```python
from build123d import *

# Parameters (mm, degrees)
F1_ANGLE = 350


with BuildPart() as f1:
    # F0 (on Top) → F1 (revolve)
    with BuildSketch(Plane.XY):
        with BuildLine():
            Line((1.2065, 2.413), (17.792, 2.413))
            Line((17.792, 2.413), (17.792, 2.7178))
            Line((17.792, 2.7178), (1.2065, 2.7178))
            ThreePointArc((1.2065, 2.7178), (0.568902, 2.981902), (0.3048, 3.6195))
            Line((0.3048, 3.6195), (0.3048, 5.3815))
            Line((0.3048, 5.3815), (0, 5.3815))
            Line((0, 5.3815), (0, 3.6195))
            ThreePointArc((0, 3.6195), (0.353376, 2.766376), (1.2065, 2.413))
        make_face()
    revolve(axis=Axis((8.896, 0, 0), (1, 0, 0)), revolution_arc=F1_ANGLE)


solid = f1.part
```
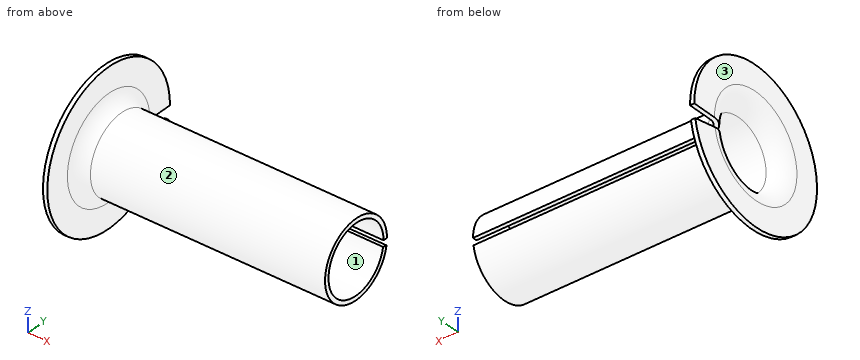
The model under review builds one solid part; all positions refer to its coordinate system, in mm. Face numbers are marked on the shaded views. Round coordinates to 2 decimals unless told otherwise and drop trailing zeros. Loops run counter-clockwise (first coordinate to the right, second up) from the corner with the lowest first, then second, coordinate; pieces in that order, holes last. Notation, with made-up numbers: (11, 43) - (44, 43) arc R31 cw to (44, 81) - close; hole circle Ø8 at (-1, 78). An arc over 180 degrees is marked (long way). Use a Markdown table: item, result. Add a question column.
Q1. Add section B-B (y = 4.5). State the section outline as (x, z) points, plus the area to 3 significant figures.
Q2. Add section D-D (z = 4.25). State the section outline as (x, y) points, plus the area to 3 significant figures.
Q3. The part is to be moulded in two halves that separate along Y. For the marked faces 1, 2 and 3, say which applies: pulls with the +Y half, pulls with the -Y half, needs draft (parallel to the pull), parting line crosses it, or undercut.
Q4. Add section C-C (x = 4.75). State the section outline as (y, z) points.
Q5. Add section A-A (y = 0). State the section outline as (x, z) points, plus the area to 3 significant figures.
Q6. For probe 1 along Z at (x, y) = (9.75, 0); probe 2 along X at (y, z) = (0.25, 4.5); probe 3 along Z at (x, y) = (10.5, 2.5), list the stretches that pass through material, from the lowest coordinate up.
Q7. Insertion check: pin 1 Ø6 at (x, z) = (13.5, -3.5) entering from +Y; pin 2 Ø1.5 at (x, y) = (9, 3.5) entering from -Z; pin 3 Ø1 at (x, y) = (7, 2) entering from -Z; pin 4 Ø6 at (x, y) = (2.5, -4) entering from +Z. Each pin has a flat end and moves straight along its axis. Give the tip position at first contact, or say it passes through.
Worked answers:
| question | item | result |
|---|---|---|
| 1 | outline | (0, -2.95) - (0.3, -2.95) - (0.3, -0.79) - (0, -0.79) - close; (0, 0) - (0.3, 0) - (0.3, 2.95) - (0, 2.95) - close |
| 1 | area | 1.56 mm² |
| 2 | outline | (0, -3.3) - (0.3, -3.3) - (0.3, 3.3) - (0, 3.3) - close |
| 2 | area | 2.01 mm² |
| 3 | face 1 | undercut |
| 3 | face 2 | parting line crosses it |
| 3 | face 3 | needs draft |
| 4 | outline | (2.38, -0.42) arc R2.41 cw (long way) to (2.41, 0) - (2.72, 0) arc R2.72 ccw (long way) to (2.68, -0.47) - close |
| 5 | outline | (0, -5.38) - (0.3, -5.38) - (0.3, -3.62) arc R0.9 cw to (1.21, -2.72) - (17.79, -2.72) - (17.79, -2.41) - (1.21, -2.41) arc R1.21 ccw to (0, -3.62) - close; (0, 3.62) arc R1.21 ccw to (1.21, 2.41) - (17.79, 2.41) - (17.79, 2.72) - (1.21, 2.72) arc R0.9 cw to (0.3, 3.62) - (0.3, 5.38) - (0, 5.38) - close |
| 5 | area | 12.2 mm² |
| 6 | probe 1 | -2.72 to -2.41, 2.41 to 2.72 |
| 6 | probe 2 | 0 to 0.3 |
| 6 | probe 3 | -1.07 to -0.44, 0 to 1.07 |
| 7 | pin 1 | y = 2.67 |
| 7 | pin 2 | through |
| 7 | pin 3 | z = -2.27 |
| 7 | pin 4 | z = 5.01 |
